```python
from build123d import *

# Parameters (mm, degrees)
F0_W     = 40
F0_H     = 31
F1_DEPTH = 5.5
F2_R     = 1
F3_W     = 34.735498
F3_H     = 18.146572
F4_DEPTH = 25


with BuildPart() as f1:
    # F0 (on Top) → F1 (new body)
    with BuildSketch(Plane.XY):
        Rectangle(F0_W, F0_H)
    extrude(amount=F1_DEPTH)

    # F2
    f2_edges = [f1.edges().sort_by_distance(p)[0] for p in [
        (20, 0, 5.5),
        (0, 15.5, 5.5),
        (-20, 0, 5.5),
        (0, -15.5, 5.5),
        (20, 0, 0),
        (0, 15.5, 0),
        (-20, 0, 0),
        (0, -15.5, 0),
        (-20, -15.5, 2.75),
        (20, -15.5, 2.75),
        (-20, 15.5, 2.75),
        (20, 15.5, 2.75),
    ]]
    fillet(f2_edges, radius=F2_R)

    # F3 (on face) → F4 (cut)
    with BuildSketch(Plane(origin=(0, 0, 0), x_dir=(1, 0, 0), z_dir=(0, 0, -1))):
        Rectangle(F3_W, F3_H)
    extrude(amount=-F4_DEPTH, mode=Mode.SUBTRACT)


solid = f1.part
```
The model under review builds one solid part; all positions refer to its coordinate system, in mm. A direction names the side the tool comes from. Round coordinates to 2 decimals unless told otherwise and drop trailing zeros. Order: outer loops, then holes, each group sorted by start corner. A loop starts at its lowest first (then second) coordinate and runs counter-clockwise, first axis right, second up. Notation, with made-up numbers: (77.25, 69.5) -> (99.25, 69.5) arc R8 ccw to (99.25, 73.5) -> close; hole circle Ø2 at (2, 80.25). An arc over 180 degrees is marked (long way). Use a Markdown table: item, result.
Q1. We need section C-C on x = 10. Write out the cut boundary in (y, z), then the cut area to 3 significant figures.
Values:
| item | result |
|---|---|
| outline | (-15.5, 1) arc R1 ccw to (-14.5, 0) -> (-9.07, 0) -> (-9.07, 5.5) -> (-14.5, 5.5) arc R1 ccw to (-15.5, 4.5) -> close; (9.07, 0) -> (14.5, 0) arc R1 ccw to (15.5, 1) -> (15.5, 4.5) arc R1 ccw to (14.5, 5.5) -> (9.07, 5.5) -> close |
| area | 69.8 mm^2 |
Q2. Tool access review of faces 4 (the flat face through (-17.368, 0, 3)), 5 (the cylindrical face through (19.699, -15.215, 2.774)): name each direction out of +Z, -Z, +X, -X, +Y, -Y from which nothing blocks a thin tool from reaching the whole face with its end or side.
Values:
| item | result |
|---|---|
| face 4 | +Z, -Z |
| face 5 | +Z, -Z, +X, -Y |
Q3. Clearance check with a flat-ended pin moving along its axis: P1, Ø12, axis at x = -6.5, y = 1.5, coming from the -Z side. State where the tip first meets the part, or that it passes through.
Values:
| item | result |
|---|---|
| P1 | passes through |
Q4. We need section A-A on y = -1. Write out the cut boundary in (x, z), then the cut area to 3 significant figures.
Values:
| item | result |
|---|---|
| outline | (-20, 1) arc R1 ccw to (-19, 0) -> (-17.37, 0) -> (-17.37, 5.5) -> (-19, 5.5) arc R1 ccw to (-20, 4.5) -> close; (17.37, 0) -> (19, 0) arc R1 ccw to (20, 1) -> (20, 4.5) arc R1 ccw to (19, 5.5) -> (17.37, 5.5) -> close |
| area | 28.1 mm^2 |
Q5. For line 1 (Y direction, x = 15, z = 3.05); line 2 (X direction, y = 4, z = 1.85); line 3 (Y direction, x = 4, z = 4.95), list the stretches that pass through material, from the lowest coordinate up.
Values:
| item | result |
|---|---|
| line 1 | y = -15.5 to -9.07, 9.07 to 15.5 |
| line 2 | x = -20 to -17.37, 17.37 to 20 |
| line 3 | y = -15.39 to -9.07, 9.07 to 15.39 |
Q6. We need section B-B on z = 3.7. Write out the cut boundary in (x, y).
Values:
| item | result |
|---|---|
| outline | (-20, -14.5) arc R1 ccw to (-19, -15.5) -> (19, -15.5) arc R1 ccw to (20, -14.5) -> (20, 14.5) arc R1 ccw to (19, 15.5) -> (-19, 15.5) arc R1 ccw to (-20, 14.5) -> close; hole (-17.37, -9.07) -> (17.37, -9.07) -> (17.37, 9.07) -> (-17.37, 9.07) -> close |
Q7. Mouldability with a two-part tool opening along X and no side actions: class faces 1 (the cylindrical face through (0.266, 15.215, 5.199)), 2 (the flat face through (20, 0, 3)), 3 (the flat face through (0, -9.073, 3)) as +X half, -X half, draft (parallel to the pull), parting line (faces both ways), or undercut.
Values:
| item | result |
|---|---|
| face 1 | draft |
| face 2 | +X half |
| face 3 | undercut |
